Check sheet for the modelled part. Datum: model origin and axes. Units: mm. A direction names the side the tool comes from. Coordinates: 2 decimals unless noted, no trailing zeros. Order: outer loops, then holes, each group sorted by start corner. A loop starts at its lowest first (then second) coordinate and runs counter-clockwise, first axis right, second up.
1. Cross-section at A-A (x = 18.9). Enter the section's corners in (y, z) (3 decimals), then the cut area to 3 significant figures.
2. Gauge pin test, flat ends, axial feed: pin 1 Ø6.5 at (y, z) = (9.5, -4.5) entering from -X; pin 2 Ø8 at (x, z) = (7, -13) entering from -Y; pin 3 Ø2 at (y, z) = (-1.5, 1) entering from -X; pin 4 Ø6 at (x, z) = (1, -5) entering from +Y. Record the tip position at first contact, or that the pin passes through.
3. Set-up check for faces 1 (the flat face through (-20.4, 13, -2)), 2 (the flat face through (46.096, 5, -15)), 3 (the flat face through (8.4, 23, 2)), 4 (the flat face through (18.12, 109.97, 2.03)): record each of +Z, -Z, +X, -X, +Y, -Y from which the full face is reachable in a straight line by a thin tool's end or side.
4. Cross-section at B-B (z = -11.5). Enter the section's corners in (x, y), then the cut area to 3 significant figures.
5. Cross-section at C-C (y = 77.5). Enter the section's corners in (x, z).
6. Thickness scan on line 1 (Y direction, x = -18.05, z = -4); line 2 (Y direction, x = 19.15, z = -4); line 3 (Z direction, x = -11, y = 71.5). Record the ranges inside material, lowest first.
7. Draft check along X on faces 5 (the flat face through (0, 17.55, 2)), 6 (the flat face through (8.4, 1, 2)), 7 (the flat face through (51.096, 5, -14)), 8 (the flat face through (47, 2.89, -10)). Enter one of: released by +X, released by -X, zero draft, split by the parting line, or undercut.
8. Cross-section at D-D (x = 43). Enter the section's corners in (y, z).
```python
from build123d import *

# Parameters (mm, degrees)
EXTRUDE_1_DEPTH     = 4
SKETCH_2_W          = 15
SKETCH_2_H          = 13.3866
CUT_EXTRUDE_1_DEPTH = 121.93395925
SKETCH_3_W          = 10
SKETCH_3_H          = 10
SKETCH_3_R          = 1.55
SKETCH_3_H_2        = 14.755
EXTRUDE_2_DEPTH     = 4
EXTRUDE_3_DEPTH     = 4
EXTRUDE_4_DEPTH     = 4
SKETCH_7_W          = 27.8
SKETCH_7_H          = 4
EXTRUDE_5_DEPTH     = 4
EXTRUDE_START       = -4
EXTRUDE_6_DEPTH     = 4
SKETCH_11_W         = 16.8
SKETCH_11_H         = 10.85
CUT_EXTRUDE_2_DEPTH = 133.52791749
CHAMFER_1_SIZE      = 2
CHAMFER_2_SIZE      = 2
SKETCH_12_W         = 12
SKETCH_12_H         = 8.55
SKETCH_12_R         = 1.25
EXTRUDE_7_DEPTH     = 4
EXTRUDE_START_2     = 4
SKETCH_13_R         = 1.25
SKETCH_13_W         = 4
SKETCH_13_H         = 8.709663749
EXTRUDE_8_DEPTH     = 4
SKETCH_14_R         = 1
CUT_EXTRUDE_3_DEPTH = 132.839329922
SKETCH_15_R         = 0.9
EXTRUDE_9_DEPTH     = 1
FILLET_1_R          = 0.9
CUT_EXTRUDE_START   = -1.7
SKETCH_16_R         = 1
CUT_EXTRUDE_4_DEPTH = 1.7
CUT_EXTRUDE_5_DEPTH = 132.839329922
SKETCH_19_W         = 5
SKETCH_19_H         = 38.5268
SKETCH_19_W_2       = 8.236887868
SKETCH_19_H_2       = 1.55
CUT_EXTRUDE_6_DEPTH = 132.839329922


with BuildPart() as part:
    # Sketch 1 → Extrude 1 (new body)
    with BuildSketch(Plane.XY):
        with BuildLine():
            Line((-16.4, -7.25), (-16.4, 119.75))
            Line((-16.4, 119.75), (16.4, 119.75))
            Line((16.4, 119.75), (16.4, -7.25))
            ThreePointArc((16.4, -7.25), (15.038046533, -10.538046533), (11.75, -11.9))
            Line((11.75, -11.9), (-11.75, -11.9))
            ThreePointArc((-11.75, -11.9), (-15.038046533, -10.538046533), (-16.4, -7.25))
        make_face()
    extrude(amount=EXTRUDE_1_DEPTH)

    # Sketch 2 → Cut-Extrude 1 (cut, through all)
    with BuildSketch(Plane(origin=(0, 0, 0), x_dir=(-1, 0, 0), z_dir=(0, 0, -1))):
        with Locations((0, 111.3567)):
            Rectangle(SKETCH_2_W, SKETCH_2_H)
    extrude(amount=-CUT_EXTRUDE_1_DEPTH, mode=Mode.SUBTRACT)

    # Sketch 3 → Extrude 2 (add)
    # profile 1 of 2: a face of its own
    with BuildSketch(Plane(origin=(0, 119.75, 0), x_dir=(1, 0, 0), z_dir=(0, 1, 0))):
        with Locations((-18.9, 15.755)):
            Rectangle(SKETCH_3_W, SKETCH_3_H)
        with Locations(Location((-18.9, 15.755, 0), (0, 0, 270))):
            Circle(SKETCH_3_R, mode=Mode.SUBTRACT)
    # profile 2 of 2: a face of its own
    with BuildSketch(Plane(origin=(0, 119.75, 0), x_dir=(1, 0, 0), z_dir=(0, 1, 0))):
        with Locations((-18.9, 3.3775)):
            Rectangle(SKETCH_3_W, SKETCH_3_H_2)
    extrude_2 = extrude(amount=-EXTRUDE_2_DEPTH)

    # Mirror 1: Extrude 2 across plane
    add(extrude_2.mirror(Plane(origin=(0, 0, 0), x_dir=(0, 0, 1), z_dir=(1, 0, 0))))

    # Sketch 6 → Extrude 4 (add)
    with BuildSketch(Plane.XY.offset(4)):
        Polygon((-16.4, 115.75), (-23.9, 115.75), (-16.4, 108.25), align=None)
        Polygon((16.4, 115.75), (16.4, 108.25), (23.9, 115.75), align=None)
    extrude(amount=-EXTRUDE_4_DEPTH)

    # Sketch 7 → Extrude 5 (add)
    with BuildSketch(Plane(origin=(0, 119.75, 0), x_dir=(1, 0, 0), z_dir=(0, 1, 0))):
        with Locations((0, 18.755)):
            Rectangle(SKETCH_7_W, SKETCH_7_H)
    extrude(amount=-EXTRUDE_5_DEPTH)



with BuildPart() as body_2:
    # Sketch 5 → Extrude 3 (new body)
    with BuildSketch(Plane(origin=(0, 2.890336251, 0), x_dir=(1, 0, 0), z_dir=(0, 1, 0))):
        Polygon((50.795757056, 9.855), (46.095757056, 9.855), (32.240757056, -4), (39.311824868, -4), (51.095757056, 7.783932188), (51.095757056, 9.855), align=None)
        with BuildLine():
            Line((50.795757056, 19.755), (46.095757056, 19.755))
            Line((46.095757056, 19.755), (46.095757056, 9.855))
            Line((46.095757056, 9.855), (50.795757056, 9.855))
            Line((50.795757056, 9.855), (50.795757056, 15.105))
            Line((50.795757056, 15.105), (49.255691264, 15.105))
            ThreePointArc((49.255691264, 15.105), (47.495757056, 15.755), (49.255691264, 16.405))
            Line((49.255691264, 16.405), (50.795757056, 16.405))
            Line((50.795757056, 16.405), (50.795757056, 19.755))
        make_face()
        with BuildLine():
            Line((51.095757056, 19.755), (50.795757056, 19.755))
            Line((50.795757056, 19.755), (50.795757056, 16.405))
            Line((50.795757056, 16.405), (49.255691264, 16.405))
            ThreePointArc((49.255691264, 16.405), (49.433822674, 16.10145764), (49.495757056, 15.755))
            ThreePointArc((49.495757056, 15.755), (49.433822674, 15.40854236), (49.255691264, 15.105))
            Line((49.255691264, 15.105), (50.795757056, 15.105))
            Line((50.795757056, 15.105), (50.795757056, 9.855))
            Line((50.795757056, 9.855), (51.095757056, 9.855))
            Line((51.095757056, 9.855), (51.095757056, 19.755))
        make_face()
    extrude(amount=EXTRUDE_3_DEPTH)


with BuildPart() as part_1:
    add(part.part)

    add(body_2.part)  # Extrude 6 merges body 2
    # Sketch 8 → Extrude 6 (add)
    with BuildSketch(Plane.XY.offset(4).offset(EXTRUDE_START)):
        with BuildLine():
            Line((26.521488617, -11.9), (39.311824868, 0.890336251))
            Line((39.311824868, 0.890336251), (39.311824868, 6.890336251))
            Line((39.311824868, 6.890336251), (16.4, 6.890336251))
            Line((16.4, 6.890336251), (16.4, -7.25))
            ThreePointArc((16.4, -7.25), (15.038046533, -10.538046533), (11.75, -11.9))
            Line((11.75, -11.9), (26.521488617, -11.9))
        make_face()
    extrude(amount=EXTRUDE_6_DEPTH)

    # Sketch 11 → Cut-Extrude 2 (cut, through all)
    with BuildSketch(Plane.XY.offset(4)):
        with Locations((0, 1.525)):
            Rectangle(SKETCH_11_W, SKETCH_11_H)
        with Locations((0, 22.975)):
            Rectangle(SKETCH_11_W, SKETCH_11_H)
    extrude(amount=-CUT_EXTRUDE_2_DEPTH, mode=Mode.SUBTRACT)

    # Chamfer 1
    chamfer_1_edges = [part_1.edges().sort_by_distance(p)[0] for p in [
        (39.311824868, 2.890336251, 2),
    ]]
    chamfer(chamfer_1_edges, length=CHAMFER_1_SIZE - 0.0001)  # a hair under: the kernel refuses the full size

    # Chamfer 2
    chamfer_2_edges = [part_1.edges().sort_by_distance(p)[0] for p in [
        (38.776240962, 2.890336251, 0),
    ]]
    chamfer(chamfer_2_edges, length=CHAMFER_2_SIZE - 0.0001)  # a hair under: the kernel refuses the full size

    # Sketch 12 → Extrude 7 (add)
    with BuildSketch(Plane.ZY.offset(16.4)):
        with Locations((-2, 13.325)):
            Rectangle(SKETCH_12_W, SKETCH_12_H)
        with Locations((-4, 12.25)):
            Circle(SKETCH_12_R, mode=Mode.SUBTRACT)
    extrude(amount=EXTRUDE_7_DEPTH)

    # Sketch 13 → Extrude 8 (add)
    # profile 1 of 2: a face of its own
    with BuildSketch(Plane(origin=(16.4, 0, 0), x_dir=(0, 0, -1), z_dir=(1, 0, 0)).offset(EXTRUDE_START_2)):
        Polygon((8, 9.890336251), (8, 15.6), (0, 15.6), (0, 6.890336251), (5, 6.890336251), align=None)
        with Locations(Location((4, 12.25, 0), (0, 0, 180))):
            Circle(SKETCH_13_R, mode=Mode.SUBTRACT)
    # profile 2 of 2: a face of its own
    with BuildSketch(Plane(origin=(16.4, 0, 0), x_dir=(0, 0, -1), z_dir=(1, 0, 0)).offset(EXTRUDE_START_2)):
        with Locations((-2, 11.245168126)):
            Rectangle(SKETCH_13_W, SKETCH_13_H)
    extrude(amount=-EXTRUDE_8_DEPTH)

    # Sketch 14 → Cut-Extrude 3 (cut, through all)
    with BuildSketch(Plane(origin=(0, 0, 0), x_dir=(-1, 0, 0), z_dir=(0, 0, -1))):
        with Locations((-5, 63.75)):
            Circle(SKETCH_14_R)
        with Locations((-5, 100.15)):
            Circle(SKETCH_14_R)
    extrude(amount=-CUT_EXTRUDE_3_DEPTH, mode=Mode.SUBTRACT)

    # Sketch 15 → Extrude 9 (add)
    with BuildSketch(Plane(origin=(0, 0, 0), x_dir=(-1, 0, 0), z_dir=(0, 0, -1))):
        with Locations(Location((-5, 95.5, 0), (0, 0, 180))):
            Circle(SKETCH_15_R)
        with Locations(Location((-5, 59.13, 0), (0, 0, 180))):
            Circle(SKETCH_15_R)
    extrude(amount=EXTRUDE_9_DEPTH)

    # Fillet 1
    fillet_1_edges = [part_1.edges().sort_by_distance(p)[0] for p in [
        (4.1, 95.5, -1),
        (4.1, 59.13, -1),
    ]]
    fillet(fillet_1_edges, radius=FILLET_1_R)

    # Sketch 16 → Cut-Extrude 4 (cut)
    # profile 1 of 2: a face of its own
    with BuildSketch(Plane.XY.offset(4).offset(CUT_EXTRUDE_START)):
        Polygon((7.05, 62.566431948), (7.05, 64.933568052), (5, 66.117136104), (2.95, 64.933568052), (2.95, 62.566431948), (5, 61.382863896), align=None)
        with Locations(Location((5, 63.75, 0), (0, 0, 180))):
            Circle(SKETCH_16_R, mode=Mode.SUBTRACT)
    # profile 2 of 2: a face of its own
    with BuildSketch(Plane.XY.offset(4).offset(CUT_EXTRUDE_START)):
        Polygon((2.95, 98.966431948), (5, 97.782863896), (7.05, 98.966431948), (7.05, 101.333568052), (5, 102.517136104), (2.95, 101.333568052), align=None)
        with Locations(Location((5, 100.15, 0), (0, 0, 180))):
            Circle(SKETCH_16_R, mode=Mode.SUBTRACT)
    extrude(amount=CUT_EXTRUDE_4_DEPTH, mode=Mode.SUBTRACT)

    # Sketch 17 → Cut-Extrude 5 (cut, symmetric)
    with BuildSketch(Plane(origin=(0, 0, 0), x_dir=(-1, 0, 0), z_dir=(0, 0, -1))):
        Polygon((-12.5, 104.35), (-16.4, 108.25), (-16.4, 41.2366), (-12.5, 45.1366), align=None)
    cut_extrude_5 = extrude(amount=CUT_EXTRUDE_5_DEPTH, both=True, mode=Mode.SUBTRACT)

    # Mirror 2: Cut-Extrude 5 across plane
    add(cut_extrude_5.mirror(Plane(origin=(0, 0, 0), x_dir=(0, 0, 1), z_dir=(1, 0, 0))), mode=Mode.SUBTRACT)

    # Sketch 19 → Cut-Extrude 6 (cut, through all)
    with BuildSketch(Plane(origin=(0, 0, 0), x_dir=(-1, 0, 0), z_dir=(0, 0, -1))):
        with Locations((2, 75.4)):
            Rectangle(SKETCH_19_W, SKETCH_19_H)
        with Locations((0, 48.825)):
            Rectangle(SKETCH_19_W_2, SKETCH_19_H_2)
    extrude(amount=-CUT_EXTRUDE_6_DEPTH, mode=Mode.SUBTRACT)


solid = part_1.part
```
Data:
1. outline: (-11.9, 0) - (6.89, 0) - (6.89, -5) - (9.89, -8) - (15.6, -8) - (15.6, 4) - (-11.9, 4) - close; (110.75, 0) - (115.75, 0) - (115.75, -14.205) - (119.75, -14.205) - (119.75, 4) - (110.75, 4) - close; (115.75, -20.755) - (119.75, -20.755) - (119.75, -17.305) - (115.75, -17.305) - close; hole circle Ø2.5 at (12.25, -4)
1. area: 277 mm2
2. pin 1: stops at x = -20.4
2. pin 2: stops at y = 115.75
2. pin 3: stops at x = -16.4
2. pin 4: passes through
3. face 1: +Z, -Z, -X, -Y
3. face 2: -Z, -X, +Y, -Y
3. face 3: +Z, -Z
3. face 4: +Z, -Z, +X
4. outline: (-23.9, 115.75) - (-13.9, 115.75) - (-13.9, 119.75) - (-23.9, 119.75) - close; (13.9, 115.75) - (23.9, 115.75) - (23.9, 119.75) - (13.9, 119.75) - close; (46.1, 2.89) - (51.1, 2.89) - (51.1, 6.89) - (46.1, 6.89) - close
4. area: 100 mm2
5. outline: (-12.5, 0) - (-4.5, 0) - (-4.5, 4) - (-12.5, 4) - close; (0.5, 0) - (12.5, 0) - (12.5, 4) - (0.5, 4) - close
6. line 1: y = 9.05 to 11, 13.5 to 17.6, 115.75 to 119.75
6. line 2: y = 6.89 to 11, 13.5 to 15.6, 115.75 to 119.75
6. line 3: z = 0 to 4
7. face 5: undercut
7. face 6: undercut
7. face 7: released by +X
7. face 8: zero draft
8. outline: (2.89, -6.76) - (6.89, -6.76) - (6.89, 0.31) - (2.89, 0.31) - close
